Verification items for this drawing (mm, ordinates from the low corner). A direction names the side the tool comes from. Give positions to 0.01 mm unless a question says otherwise; leave off trailing zeros. Write each loop counter-clockwise with the first axis right and the second up, starting at its lowest first coordinate (ties: lowest second). Pieces come first, ordered by that corner, then holes. Notation, with made-up numbers: M 52.5,-31.5 L 78.5,-31.5 A4 ccw 78.5,-26.5 Z; hole C 34.5,37 d4. An arc over 180 degrees is marked long. Use one line per item in the form item = value. Start each with the question number.
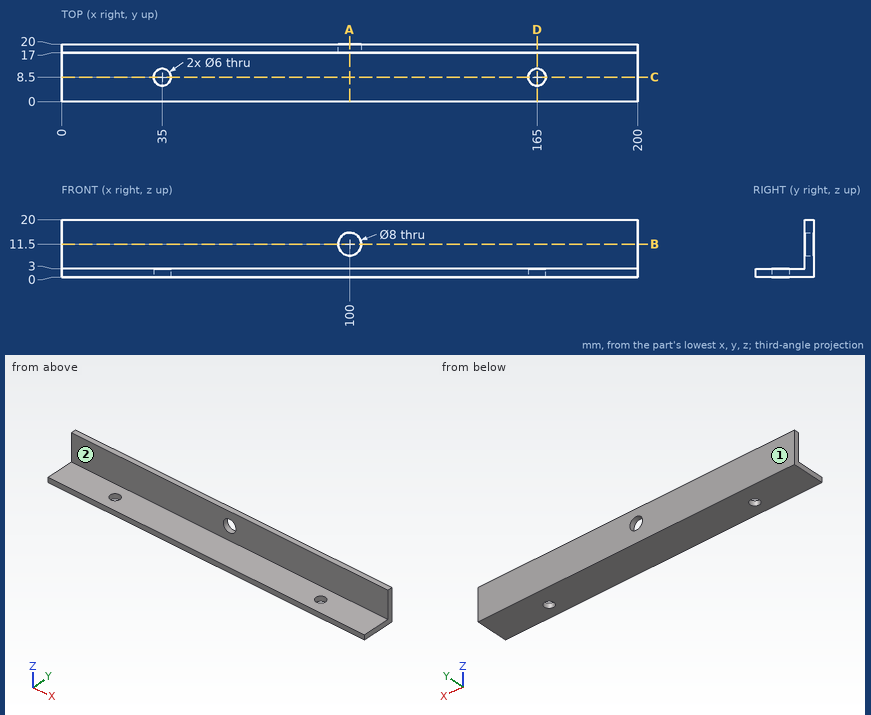
(1) Thickness scan on probe 1 along X at (y, z) = (8.5, 1.6); probe 2 along Y at (x, z) = (35, 2.3); probe 3 along Z at (x, y) = (100, 18.75). Record the ranges inside material, lowest first. Write a range as [from, to].
(2) Sectioned sample at B-B, the plane z = 11.5. Record the boundary of the cut face in (x, y), plus the area to 3 significant figures.
(3) Depth check by flat-ended pin: pin 1 (5 mm diameter, centred on x = 156.5, z = 7, fed in from -Y); pin 2 (5.5 mm diameter, centred on x = 35, y = 8.5, fed in from -Z); pin 3 (5 mm diameter, centred on x = 87, y = 5.5, fed in from +Z). Enter the tip coordinate at first touch or a pass-through.
(4) Tool access check on the marked faces 1 and 2. Record the directions out of +Z, -Z, +X, -X, +Y, -Y that give a thin tool (end or side, any length) a straight path to the whole face; none if there is none.
(5) Sectioned sample at C-C, the plane y = 8.5. Record the boundary of the cut face in (x, z), plus the area to 3 significant figures.
(6) Sectioned sample at D-D, the plane x = 165. Record the boundary of the cut face in (y, z), plus the area to 3 significant figures.
(7) Sectioned sample at A-A, the plane x = 100. Record the boundary of the cut face in (y, z).
Numbers:
q1.probe_1 = [0, 32], [38, 162], [168, 200]
q1.probe_2 = [0, 5.5], [11.5, 20]
q1.probe_3 = [0, 7.5], [15.5, 20]
q2.outline = M 0,17 L 96,17 L 96,20 L 0,20 Z; M 104,17 L 200,17 L 200,20 L 104,20 Z
q2.area = 576 mm2
q3.pin_1 = 17
q3.pin_2 = through
q3.pin_3 = 3
q4.face_1 = +Z, -Z, +X, -X, +Y
q4.face_2 = +Z, +X, -X, -Y
q5.outline = M 0,0 L 32,0 L 32,3 L 0,3 Z; M 38,0 L 162,0 L 162,3 L 38,3 Z; M 168,0 L 200,0 L 200,3 L 168,3 Z
q5.area = 564 mm2
q6.outline = M 0,0 L 5.5,0 L 5.5,3 L 0,3 Z; M 11.5,0 L 20,0 L 20,20 L 17,20 L 17,3 L 11.5,3 Z
q6.area = 93.0 mm2
q7.outline = M 0,0 L 20,0 L 20,7.5 L 17,7.5 L 17,3 L 0,3 Z; M 17,15.5 L 20,15.5 L 20,20 L 17,20 Z
